Read the model definition and answer for the solid it produces. Units are mm, in the model's axes. A direction names the side the tool comes from. Round coordinates to 2 decimals unless told otherwise and drop trailing zeros. Order: outer loops, then holes, each group sorted by start corner. A loop starts at its lowest first (then second) coordinate and runs counter-clockwise, first axis right, second up. Notation, with made-up numbers: (-19, -39.5) -> (37, -39.5) arc R15 cw to (37, -10.5) -> close; hole circle Ø8 at (68, 24). An arc over 180 degrees is marked (long way). One line per item, written item: value. Start each with the question number.
1. The mould has two halves that part along Z. Classify faces 5 (the face through (20.2, 40, 10)), 6 (the face through (40, -10, -23.2)), 7 (the face through (-20.4, 10, -40)), 8 (the face through (55.613, 5.986, -8.754)): released by +Z, released by -Z, zero draft, split by the parting line, or undercut.
2. Section A-A (x = -4.5) is taken. Give the vertices of the cut face in (y, z), then the cut area to 3 significant figures.
3. Section C-C (z = 14) is taken. Give the vertices of the cut face in (x, y), then the cut area to 3 significant figures.
4. Consider line 1 (Z direction, x = 6.8, y = 10); line 2 (X direction, y = 35, z = 19); line 3 (Y direction, x = 1.8, z = -50). Determine where each line is inside the solid, lowest interval first.
5. Section D-D (x = 50) is taken. Give the vertices of the cut face in (y, z).
6. Section B-B (y = 50) is taken. Give the vertices of the cut face in (x, z), then the cut area to 3 significant figures.
7. Flat-ended cylindrical pins translate along their axes: pin 1 Ø5 at (y, z) = (25.5, -8.5) entering from +X; pin 2 Ø8 at (x, z) = (-14, -40.5) entering from +Y; pin 3 Ø16.5 at (y, z) = (44, -10.5) entering from -X; pin 4 Ø10 at (x, z) = (46.5, 9) entering from +Y. Find the tip coordinate at first contact, or state that the pin passes through.
8. For faces 1 (the face through (-2, -2, -20.3)), 2 (the face through (23.2, 40, 10)), 3 (the face through (-10, 23.2, -40)), 4 (the face through (6.49, 13.77, -47.11)), determine the directions among +Z, -Z, +X, -X, +Y, -Y from which every point of the face is accessible in a straight line to the end or side of a thin tool.
from build123d import *

# Parameters (mm, degrees)
SKETCH1_W           = 20
SKETCH1_H           = 20
BOSS_EXTRUDE1_DEPTH = 20
SKETCH2_W           = 40
SKETCH2_H           = 20
BOSS_EXTRUDE2_DEPTH = 5
BOSS_EXTRUDE3_DEPTH = 3
BOSS_EXTRUDE4_START = -20
BOSS_EXTRUDE4_DEPTH = 3
SKETCH4_R           = 4.75
SKETCH4_R_2         = 2.75
BOSS_EXTRUDE5_DEPTH = 1
SKETCH4_3_R         = 2.75
CUT_EXTRUDE1_DEPTH  = 66
SKETCH4_4_R         = 5.75
SKETCH4_4_R_2       = 4.75
BOSS_EXTRUDE6_DEPTH = 2
BOSS_EXTRUDE7_START = -20.3
BOSS_EXTRUDE7_DEPTH = 39.7
CIRPATTERN1_COUNT   = 3


with BuildPart() as part:
    # Sketch1 → Boss-Extrude1 (new body)
    with BuildSketch(Plane(origin=(0, 0, 0), x_dir=(1, 0, 0), z_dir=(0, 1, 0))):
        with Locations((10, 10)):
            Rectangle(SKETCH1_W, SKETCH1_H)
    extrude(amount=BOSS_EXTRUDE1_DEPTH)

    # Sketch2 → Boss-Extrude2 (add)
    with BuildSketch(Plane(origin=(0, 0, 0), x_dir=(1, 0, 0), z_dir=(0, 1, 0))):
        with Locations((40, 10)):
            Rectangle(SKETCH2_W, SKETCH2_H)
    boss_extrude2 = extrude(amount=BOSS_EXTRUDE2_DEPTH)

    # Sketch3 → Boss-Extrude3 (add)
    with BuildSketch(Plane.XY):
        Polygon((20, 5), (20, 20), (60, 5), align=None)
    boss_extrude3 = extrude(amount=-BOSS_EXTRUDE3_DEPTH)

    # Sketch3<2> → Boss-Extrude4 (add)
    with BuildSketch(Plane.XY.offset(BOSS_EXTRUDE4_START)):
        Polygon((20, 5), (20, 20), (60, 5), align=None)
    boss_extrude4 = extrude(amount=BOSS_EXTRUDE4_DEPTH)

    # Sketch4 → Boss-Extrude5 (add)
    with BuildSketch(Plane(origin=(0, 5, 0), x_dir=(1, 0, 0), z_dir=(0, 1, 0))):
        with Locations(Location((50, 10, 0), (0, 0, 90))):
            Circle(SKETCH4_R)
        with Locations(Location((50, 10, 0), (0, 0, 270))):
            Circle(SKETCH4_R_2, mode=Mode.SUBTRACT)
    boss_extrude5 = extrude(amount=BOSS_EXTRUDE5_DEPTH)

    # Sketch4<3> → Cut-Extrude1 (cut, through all)
    with BuildSketch(Plane(origin=(0, 5, 0), x_dir=(1, 0, 0), z_dir=(0, 1, 0))):
        with Locations(Location((50, 10, 0), (0, 0, 270))):
            Circle(SKETCH4_3_R)
    cut_extrude1 = extrude(amount=-CUT_EXTRUDE1_DEPTH, mode=Mode.SUBTRACT)

    # Sketch4<4> → Boss-Extrude6 (add)
    with BuildSketch(Plane(origin=(0, 5, 0), x_dir=(1, 0, 0), z_dir=(0, 1, 0))):
        with Locations(Location((50, 10, 0), (0, 0, 90))):
            Circle(SKETCH4_4_R)
        with Locations(Location((50, 10, 0), (0, 0, 270))):
            Circle(SKETCH4_4_R_2, mode=Mode.SUBTRACT)
    boss_extrude6 = extrude(amount=BOSS_EXTRUDE6_DEPTH)

    # Sketch5 → Boss-Extrude7 (add)
    with BuildSketch(Plane.ZY.offset(BOSS_EXTRUDE7_START)):
        Polygon((-20.2, -20.4), (-20.2, 0), (-20, 0), (-20, 3), (-23.2, 3), (-23.2, -23.4), (3.2, -23.4), (3.2, 3), (0, 3), (0, 0), (0.2, 0), (0.2, -20.4), align=None)
    boss_extrude7 = extrude(amount=-BOSS_EXTRUDE7_DEPTH)

    # CirPattern1: Boss-Extrude2, Boss-Extrude3, Boss-Extrude4, Boss-Extrude5, Cut-Extrude1, Boss-Extrude6, Boss-Extrude7 ×3 about axis
    cirpattern1_axis = Axis((0, 0, 0), (0.5773502691896256, 0.5773502691896258, -0.5773502691896258))
    add([boss_extrude2.rotate(cirpattern1_axis, i * 360 / CIRPATTERN1_COUNT) for i in range(1, CIRPATTERN1_COUNT)])
    add([boss_extrude3.rotate(cirpattern1_axis, i * 360 / CIRPATTERN1_COUNT) for i in range(1, CIRPATTERN1_COUNT)])
    add([boss_extrude4.rotate(cirpattern1_axis, i * 360 / CIRPATTERN1_COUNT) for i in range(1, CIRPATTERN1_COUNT)])
    add([boss_extrude5.rotate(cirpattern1_axis, i * 360 / CIRPATTERN1_COUNT) for i in range(1, CIRPATTERN1_COUNT)])
    add([cut_extrude1.rotate(cirpattern1_axis, i * 360 / CIRPATTERN1_COUNT) for i in range(1, CIRPATTERN1_COUNT)], mode=Mode.SUBTRACT)
    add([boss_extrude6.rotate(cirpattern1_axis, i * 360 / CIRPATTERN1_COUNT) for i in range(1, CIRPATTERN1_COUNT)])
    add([boss_extrude7.rotate(cirpattern1_axis, i * 360 / CIRPATTERN1_COUNT) for i in range(1, CIRPATTERN1_COUNT)])

    # SurfaceCut1
    split(bisect_by=Plane(origin=(3.464101615, 3.464101615, -3.464101615), x_dir=(0.8164965809277263, -0.40824829046386285, 0.40824829046386285), z_dir=(-0.5773502691896255, -0.5773502691896256, 0.5773502691896262)), keep=Keep.BOTTOM)


solid = part.part
Answer:
1. face 5: undercut
1. face 6: released by -Z
1. face 7: zero draft
1. face 8: undercut
2. outline: (-3.2, -60) -> (-0.2, -60) -> (-0.2, -20.3) -> (-3.2, -20.3) -> close; (20.2, -60) -> (23.2, -60) -> (23.2, -20.3) -> (20.2, -20.3) -> close
2. area: 238 mm^2
3. outline: (-3.2, 27.59) -> (-0.2, 24.59) -> (-0.2, 60) -> (-3.2, 60) -> close; (20.2, 20.3) -> (23.2, 20.3) -> (23.2, 60) -> (20.2, 60) -> close
3. area: 221 mm^2
4. line 1: -55.75 to -54.75, -45.25 to -44.25, -20 to 0
4. line 2: -3.2 to -0.2, 20.2 to 23.2
4. line 3: -3.2 to 7.25, 12.75 to 23.2
5. outline: (-23.4, -23.2) -> (3, -23.2) -> (3, -20) -> (8.75, -20) -> (8.75, -17) -> (5, -17) -> (5, -15.75) -> (7, -15.75) -> (7, -14.75) -> (6, -14.75) -> (6, -12.75) -> (0, -12.75) -> (0, -20.2) -> (-20.4, -20.2) -> (-20.4, 0.2) -> (0, 0.2) -> (0, -7.25) -> (6, -7.25) -> (6, -5.25) -> (7, -5.25) -> (7, -4.25) -> (5, -4.25) -> (5, -3) -> (8.75, -3) -> (8.75, 0) -> (3, 0) -> (3, 3.2) -> (-23.4, 3.2) -> close
6. outline: (-3.2, -3) -> (0, -3) -> (0, -8.75) -> (3, -8.75) -> (3, -5) -> (4.25, -5) -> (4.25, -7) -> (5.25, -7) -> (5.25, -6) -> (7.25, -6) -> (7.25, 0) -> (-0.2, 0) -> (-0.2, 20.4) -> (20.2, 20.4) -> (20.2, 0) -> (12.75, 0) -> (12.75, -6) -> (14.75, -6) -> (14.75, -7) -> (15.75, -7) -> (15.75, -5) -> (17, -5) -> (17, -8.75) -> (20, -8.75) -> (20, -3) -> (23.2, -3) -> (23.2, 23.4) -> (-3.2, 23.4) -> close
6. area: 324 mm^2
7. pin 1: x = 20
7. pin 2: y = 23.2
7. pin 3: x = -3.2
7. pin 4: through
8. face 1: +Z, -X, -Y
8. face 2: +Z, -Z, +X, +Y
8. face 3: -Z, +X, -X, +Y
8. face 4: +X
